The listing builds one solid part. Answer for the finished solid, in the listing's coordinates (mm). A direction names the side the tool comes from. Coordinates: 2 decimals unless noted, no trailing zeros. Order: outer loops, then holes, each group sorted by start corner. A loop starts at its lowest first (then second) coordinate and runs counter-clockwise, first axis right, second up. Notation, with made-up numbers: (27.5, -16) -> (42.5, -16) arc R20 cw to (42.5, -3) -> close; hole circle Ø8 at (74.5, 5.5). An arc over 180 degrees is marked (long way). Write item = value, one per line. Start each with the question number.
```python
from build123d import *

# Parameters (mm, degrees)
F8_W      = 22.225
F8_H      = 76.2
F9_DEPTH  = 3.175
F0_W      = 22.225
F0_H      = 57.15
F10_DEPTH = 12.7
F1_R      = 2.38125
F2_DEPTH  = 3.175
F3_W      = 3.175
F3_H      = 49.2125
F3_H_2    = 52.3875
F4_DEPTH  = 22.225
F5_R      = 1.58749
F6_R      = 7.93749
F7_R      = 4.76249


# Not quite as in the source:
# - a fillet or chamfer is up to 0.001 mm smaller than in the source, because OpenCascade refuses the exact size


with BuildPart() as f9:
    # F8 (on Front) → F9 (new body)
    with BuildSketch(Plane.XZ):
        Rectangle(F8_W, F8_H)
    extrude(amount=F9_DEPTH)

    # F0 (on face) → F10 (join)
    with BuildSketch(Plane.XZ.offset(3.175)):
        with Locations((0, 9.525)):
            Rectangle(F0_W, F0_H)
    extrude(amount=F10_DEPTH)

    # F1 (on face) → F2 (cut, through all)
    with BuildSketch(Plane.XZ.offset(3.175)):
        with Locations((0, -31.75)):
            Circle(F1_R)
    extrude(amount=-F2_DEPTH, mode=Mode.SUBTRACT)

    # F3 (on face) → F4 (cut, through all)
    with BuildSketch(Plane.YZ.offset(11.1125)):
        with Locations((-11.1125, 8.73125)):
            Rectangle(F3_W, F3_H)
        with Locations((-4.7625, 7.14375)):
            Rectangle(F3_W, F3_H_2)
    extrude(amount=-F4_DEPTH, mode=Mode.SUBTRACT)

    # F5 (radius 1.5875 in the source; OpenCascade refuses exactly that, so slightly less here)
    f5_edges = [f9.edges().sort_by_distance(p)[0] for p in [
        (0, -12.7, 33.3375),
        (0, -6.35, 33.3375),
        (0, -9.525, 33.3375),
        (0, -3.175, 33.3375),
        (0, -12.7, -15.875),
        (0, -9.525, -15.875),
        (0, 0, -38.1),
        (0, -3.175, -38.1),
    ]]
    fillet(f5_edges, radius=F5_R)

    # F6 (radius 7.9375 in the source; OpenCascade refuses exactly that, so slightly less here)
    f6_edges = [f9.edges().sort_by_distance(p)[0] for p in [
        (0, -15.875, 38.1),
        (0, 0, 38.1),
    ]]
    fillet(f6_edges, radius=F6_R)

    # F7 (radius 4.7625 in the source; OpenCascade refuses exactly that, so slightly less here)
    f7_edges = [f9.edges().sort_by_distance(p)[0] for p in [
        (0, -15.875, -19.05),
        (0, -6.35, -19.05),
    ]]
    fillet(f7_edges, radius=F7_R)


solid = f9.part
```
Item 1: Section A-A, the plane x = 0 is taken. Give the number of separate pieces and of enclosed holes in the cut face, then the cut area to 3 significant figures.
Item 2: Each of these flat-tipped pins is pushed along its axis until it touches: pin 1 (8 mm diameter, centred on x = -8, z = -28.5, fed in from -Y) (3 decimals); pin 2 (4.5 mm diameter, centred on x = 0, z = -31.75, fed in from +Y); pin 3 (5 mm diameter, centred on x = -1.5, y = -3.5, fed in from +Z); pin 4 (3 mm diameter, centred on x = -8.5, y = -2.5, fed in from +Z). Where does it stop, or does it pass through?
Item 3: Which of the six approach directions +Z, -Z, +X, -X, +Y, -Y give full straight-line access (tool end or side, diameter ignored) to faces 4 (the cylindrical face through (0.16, -2.26, 35.71)), 5 (the flat face through (0, -3.175, -2)), 6 (the cylindrical face through (-0.16, -9.98, -15.4))?
Item 4: Section C-C, the plane z = -31.75 is taken. Give the vertices of the cut face in (x, y) (1 decimal).
Item 5: Consider probe 1 along Y at (x, z) = (0.5, -5.5) (3 decimals); probe 2 along Y at (x, z) = (5, -25.5) (3 decimals); probe 3 along Z at (x, y) = (0, -0.7). Determine where each line is inside the solid, lowest interval first.
Item 6: For a pull along Z with two mould halves and no side action, classify faces 1 (the cylindrical face through (-0.156, -12.223, -15.422)), 2 (the cylindrical face through (0.156, -13.488, 35.837)), 3 (the cylindrical face through (0.16, -0.48, -37.65)) as pulls with the +Z half, pulls with the -Z half, needs draft (parallel to the pull), parting line crosses it, or undercut.
A:
q1.separate_pieces = 2
q1.enclosed_holes = 1
q1.area = 595 mm^2
q2.pin_1 = -3.175
q2.pin_2 = through
q2.pin_3 = 37.86
q2.pin_4 = 37.05
q3.face_4 = +Z, +X, -X, +Y
q3.face_5 = -Z, +X, -X
q3.face_6 = +X, -X
q4.outline = (-11.1, -3.2) -> (-2.4, -3.2) -> (-2.4, 0) -> (-11.1, 0) -> close; (2.4, -3.2) -> (11.1, -3.2) -> (11.1, 0) -> (2.4, 0) -> close
q5.probe_1 = -15.875 to -12.7, -9.525 to -6.35, -3.175 to 0
q5.probe_2 = -3.175 to 0
q5.probe_3 = -37.83 to -34.13, -29.37 to 33.42
q6.face_1 = undercut
q6.face_2 = pulls with the +Z half
q6.face_3 = pulls with the -Z half
